Answer from the drawing. Dimensions are ordinates in mm from the lowest x, y and z of the part. Round coordinates to 2 decimals unless told otherwise and drop trailing zeros. Loops run counter-clockwise (first coordinate to the right, second up) from the corner with the lowest first, then second, coordinate; pieces in that order, holes last. Notation, with made-up numbers: (7, 18) - (24, 18) arc R20 cw to (24, 48) - close; hole circle Ø5 at (1.5, 23.25). An arc over 180 degrees is marked (long way). Write item = value, one per line. Start each with the question number.
1) For a pull along Z with two mould halves and no side action, classify the marked faces 1, 2, 3 and 4 as released by +Z, released by -Z, zero draft, split by the parting line, or undercut.
2) Given pin 1 Ø1.9 at (x, z) = (4, 22) entering from -Y, flat-ended and moving along its own axis, determine where the tip first touches the part or whether it passes through.
3) Section C-C, the plane y = 0.25 is taken. Determine the outline of the cut face in (x, z), and give its area (3 significant figures).
4) Straight lines are drawn through the part: line 1 along Z through (x, y) = (4, 0.85); line 2 along X through (y, z) = (0.75, 22); line 3 along Z through (x, y) = (5, 1.6). For each, find the intervals that lie inside material, in ascending order.
5) Section A-A, the plane z = 22 is taken. Determine the outline of the cut face in (x, y).
6) Section D-D, the plane z = 13 is taken. Determine the outline of the cut face in (x, y), and give its area (3 significant figures).
7) Section B-B, the plane x = 4 is taken. Determine the outline of the cut face in (y, z), and give its area (3 significant figures).
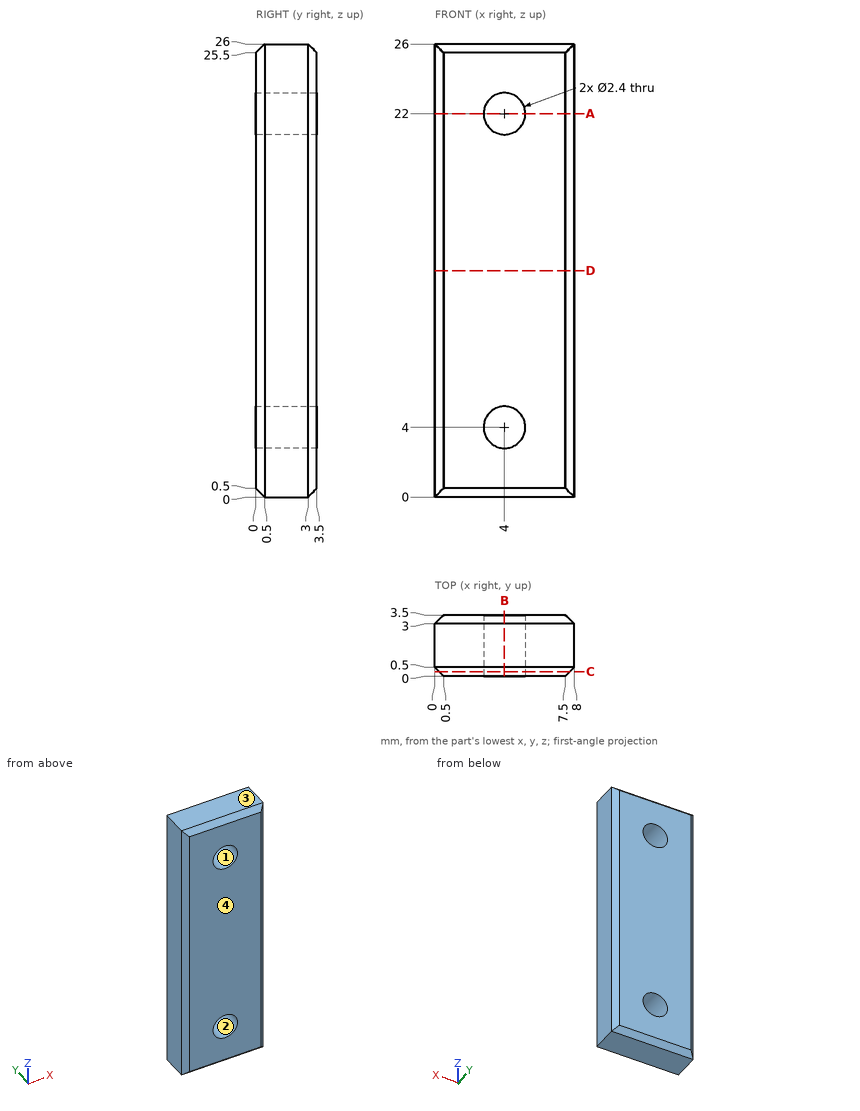
Geometry check:
q1.face_1 = undercut
q1.face_2 = undercut
q1.face_3 = released by +Z
q1.face_4 = zero draft
q2.pin_1 = through
q3.outline = (0.25, 0.25) - (7.75, 0.25) - (7.75, 25.75) - (0.25, 25.75) - close; hole circle Ø2.4 at (4, 4); hole circle Ø2.4 at (4, 22)
q3.area = 182 mm2
q4.line_1 = 0 to 2.8, 5.2 to 20.8, 23.2 to 26
q4.line_2 = 0 to 2.8, 5.2 to 8
q4.line_3 = 0 to 3.34, 4.66 to 21.34, 22.66 to 26
q5.outline = (0, 0.5) - (0.5, 0) - (2.8, 0) - (2.8, 3.5) - (0.5, 3.5) - (0, 3) - close; (5.2, 0) - (7.5, 0) - (8, 0.5) - (8, 3) - (7.5, 3.5) - (5.2, 3.5) - close
q6.outline = (0, 0.5) - (0.5, 0) - (7.5, 0) - (8, 0.5) - (8, 3) - (7.5, 3.5) - (0.5, 3.5) - (0, 3) - close
q6.area = 27.5 mm2
q7.outline = (0, 0.5) - (0.5, 0) - (3, 0) - (3.5, 0.5) - (3.5, 2.8) - (0, 2.8) - close; (0, 5.2) - (3.5, 5.2) - (3.5, 20.8) - (0, 20.8) - close; (0, 23.2) - (3.5, 23.2) - (3.5, 25.5) - (3, 26) - (0.5, 26) - (0, 25.5) - close
q7.area = 73.7 mm2
